Model file for the job. Use its own axes, mm. A direction names the side the tool comes from. Coordinates: 2 decimals unless noted, no trailing zeros. Loops run counter-clockwise (first coordinate to the right, second up) from the corner with the lowest first, then second, coordinate; pieces in that order, holes last. Notation, with made-up numbers: (7, -30) - (33, -30) arc R16 ccw to (33, -22) - close; hole circle Ø5 at (85, 72). An arc over 180 degrees is marked (long way). Write each question's results on one line, items separated by ' | '. Start each with the question number.
```python
from build123d import *

# Parameters (mm, degrees)
F0_W     = 44.45
F0_H     = 228.6
F1_DEPTH = 6.35
F3_DEPTH = 44.45
F5_DEPTH = 12.7
F7_DEPTH = 25.4


with BuildPart() as f1:
    # F0 (on Top) → F1 (new body)
    with BuildSketch(Plane.XY):
        with Locations((0, -114.3)):
            Rectangle(F0_W, F0_H)
    extrude(amount=-F1_DEPTH)

    # F2 (on face) → F3 (join)
    with BuildSketch(Plane.YZ.offset(22.225)):
        with BuildLine():
            ThreePointArc((-21.82495, 0), (-21.592466, -0.561266), (-21.0312, -0.79375))
            Line((-21.0312, -0.79375), (-21.0312, 0))
            Line((-21.0312, 0), (-21.82495, 0))
        make_face()
        with BuildLine():
            Line((-21.0312, 0), (-21.0312, -0.79375))
            ThreePointArc((-21.0312, -0.79375), (-20.469934, -0.561266), (-20.23745, 0))
            Line((-20.23745, 0), (-21.0312, 0))
        make_face()
        with BuildLine():
            ThreePointArc((-41.66235, 0), (-41.429866, -0.561266), (-40.8686, -0.79375))
            Line((-40.8686, -0.79375), (-40.8686, 0))
            Line((-40.8686, 0), (-41.66235, 0))
        make_face()
        with BuildLine():
            Line((-40.8686, 0), (-40.8686, -0.79375))
            ThreePointArc((-40.8686, -0.79375), (-40.307334, -0.561266), (-40.07485, 0))
            Line((-40.07485, 0), (-40.8686, 0))
        make_face()
        with BuildLine():
            ThreePointArc((-60.40755, 0), (-60.175066, -0.561266), (-59.6138, -0.79375))
            Line((-59.6138, -0.79375), (-59.6138, 0))
            Line((-59.6138, 0), (-60.40755, 0))
        make_face()
        with BuildLine():
            Line((-59.6138, 0), (-59.6138, -0.79375))
            ThreePointArc((-59.6138, -0.79375), (-59.052534, -0.561266), (-58.82005, 0))
            Line((-58.82005, 0), (-59.6138, 0))
        make_face()
        with BuildLine():
            ThreePointArc((-78.08595, 0), (-77.853466, -0.561266), (-77.2922, -0.79375))
            Line((-77.2922, -0.79375), (-77.2922, 0))
            Line((-77.2922, 0), (-78.08595, 0))
        make_face()
        with BuildLine():
            Line((-77.2922, 0), (-77.2922, -0.79375))
            ThreePointArc((-77.2922, -0.79375), (-76.730934, -0.561266), (-76.49845, 0))
            Line((-76.49845, 0), (-77.2922, 0))
        make_face()
        with BuildLine():
            ThreePointArc((-94.77375, 0), (-94.541266, -0.561266), (-93.98, -0.79375))
            Line((-93.98, -0.79375), (-93.98, 0))
            Line((-93.98, 0), (-94.77375, 0))
        make_face()
        with BuildLine():
            Line((-93.98, 0), (-93.98, -0.79375))
            ThreePointArc((-93.98, -0.79375), (-93.418734, -0.561266), (-93.18625, 0))
            Line((-93.18625, 0), (-93.98, 0))
        make_face()
        with BuildLine():
            ThreePointArc((-110.52175, 0), (-110.289266, -0.561266), (-109.728, -0.79375))
            Line((-109.728, -0.79375), (-109.728, 0))
            Line((-109.728, 0), (-110.52175, 0))
        make_face()
        with BuildLine():
            Line((-109.728, 0), (-109.728, -0.79375))
            ThreePointArc((-109.728, -0.79375), (-109.166734, -0.561266), (-108.93425, 0))
            Line((-108.93425, 0), (-109.728, 0))
        make_face()
        with BuildLine():
            ThreePointArc((-125.40615, 0), (-125.173666, -0.561266), (-124.6124, -0.79375))
            Line((-124.6124, -0.79375), (-124.6124, 0))
            Line((-124.6124, 0), (-125.40615, 0))
        make_face()
        with BuildLine():
            Line((-124.6124, 0), (-124.6124, -0.79375))
            ThreePointArc((-124.6124, -0.79375), (-124.051134, -0.561266), (-123.81865, 0))
            Line((-123.81865, 0), (-124.6124, 0))
        make_face()
        with BuildLine():
            ThreePointArc((-139.42695, 0), (-139.194466, -0.561266), (-138.6332, -0.79375))
            Line((-138.6332, -0.79375), (-138.6332, 0))
            Line((-138.6332, 0), (-139.42695, 0))
        make_face()
        with BuildLine():
            Line((-138.6332, 0), (-138.6332, -0.79375))
            ThreePointArc((-138.6332, -0.79375), (-138.071934, -0.561266), (-137.83945, 0))
            Line((-137.83945, 0), (-138.6332, 0))
        make_face()
        with BuildLine():
            ThreePointArc((-152.68575, 0), (-152.453266, -0.561266), (-151.892, -0.79375))
            Line((-151.892, -0.79375), (-151.892, 0))
            Line((-151.892, 0), (-152.68575, 0))
        make_face()
        with BuildLine():
            Line((-151.892, 0), (-151.892, -0.79375))
            ThreePointArc((-151.892, -0.79375), (-151.330734, -0.561266), (-151.09825, 0))
            Line((-151.09825, 0), (-151.892, 0))
        make_face()
        with BuildLine():
            ThreePointArc((-165.18255, 0), (-164.950066, -0.561266), (-164.3888, -0.79375))
            Line((-164.3888, -0.79375), (-164.3888, 0))
            Line((-164.3888, 0), (-165.18255, 0))
        make_face()
        with BuildLine():
            Line((-164.3888, 0), (-164.3888, -0.79375))
            ThreePointArc((-164.3888, -0.79375), (-163.827534, -0.561266), (-163.59505, 0))
            Line((-163.59505, 0), (-164.3888, 0))
        make_face()
        with BuildLine():
            ThreePointArc((-176.96815, 0), (-176.735666, -0.561266), (-176.1744, -0.79375))
            Line((-176.1744, -0.79375), (-176.1744, 0))
            Line((-176.1744, 0), (-176.96815, 0))
        make_face()
        with BuildLine():
            Line((-176.1744, 0), (-176.1744, -0.79375))
            ThreePointArc((-176.1744, -0.79375), (-175.613134, -0.561266), (-175.38065, 0))
            Line((-175.38065, 0), (-176.1744, 0))
        make_face()
        with BuildLine():
            ThreePointArc((-188.11875, 0), (-187.886266, -0.561266), (-187.325, -0.79375))
            Line((-187.325, -0.79375), (-187.325, 0))
            Line((-187.325, 0), (-188.11875, 0))
        make_face()
        with BuildLine():
            Line((-187.325, 0), (-187.325, -0.79375))
            ThreePointArc((-187.325, -0.79375), (-186.763734, -0.561266), (-186.53125, 0))
            Line((-186.53125, 0), (-187.325, 0))
        make_face()
        with BuildLine():
            Line((-40.8686, 0), (-40.07485, 0))
            ThreePointArc((-40.07485, 0), (-40.8686, 0.79375), (-41.66235, 0))
            Line((-41.66235, 0), (-40.8686, 0))
        make_face()
        with BuildLine():
            Line((-59.6138, 0), (-58.82005, 0))
            ThreePointArc((-58.82005, 0), (-59.6138, 0.79375), (-60.40755, 0))
            Line((-60.40755, 0), (-59.6138, 0))
        make_face()
        with BuildLine():
            Line((-77.2922, 0), (-76.49845, 0))
            ThreePointArc((-76.49845, 0), (-77.2922, 0.79375), (-78.08595, 0))
            Line((-78.08595, 0), (-77.2922, 0))
        make_face()
        with BuildLine():
            Line((-93.98, 0), (-93.18625, 0))
            ThreePointArc((-93.18625, 0), (-93.98, 0.79375), (-94.77375, 0))
            Line((-94.77375, 0), (-93.98, 0))
        make_face()
        with BuildLine():
            Line((-109.728, 0), (-108.93425, 0))
            ThreePointArc((-108.93425, 0), (-109.728, 0.79375), (-110.52175, 0))
            Line((-110.52175, 0), (-109.728, 0))
        make_face()
        with BuildLine():
            Line((-124.6124, 0), (-123.81865, 0))
            ThreePointArc((-123.81865, 0), (-124.6124, 0.79375), (-125.40615, 0))
            Line((-125.40615, 0), (-124.6124, 0))
        make_face()
        with BuildLine():
            Line((-138.6332, 0), (-137.83945, 0))
            ThreePointArc((-137.83945, 0), (-138.6332, 0.79375), (-139.42695, 0))
            Line((-139.42695, 0), (-138.6332, 0))
        make_face()
        with BuildLine():
            Line((-151.892, 0), (-151.09825, 0))
            ThreePointArc((-151.09825, 0), (-151.892, 0.79375), (-152.68575, 0))
            Line((-152.68575, 0), (-151.892, 0))
        make_face()
        with BuildLine():
            Line((-164.3888, 0), (-163.59505, 0))
            ThreePointArc((-163.59505, 0), (-164.3888, 0.79375), (-165.18255, 0))
            Line((-165.18255, 0), (-164.3888, 0))
        make_face()
        with BuildLine():
            Line((-176.1744, 0), (-175.38065, 0))
            ThreePointArc((-175.38065, 0), (-176.1744, 0.79375), (-176.96815, 0))
            Line((-176.96815, 0), (-176.1744, 0))
        make_face()
        with BuildLine():
            Line((-187.325, 0), (-186.53125, 0))
            ThreePointArc((-186.53125, 0), (-187.325, 0.79375), (-188.11875, 0))
            Line((-188.11875, 0), (-187.325, 0))
        make_face()
        with BuildLine():
            Line((-21.82495, 0), (-21.0312, 0))
            Line((-21.0312, 0), (-20.23745, 0))
            ThreePointArc((-20.23745, 0), (-21.0312, 0.79375), (-21.82495, 0))
        make_face()
    extrude(amount=-F3_DEPTH)

    # F4 (on Top) → F5 (cut, symmetric)
    with BuildSketch(Plane.XY):
        Polygon((22.286486, 0), (14.2875, 0), (22.286486, -228.6), align=None)
        Polygon((-14.2875, 0), (-22.363186, 0), (-22.363186, -228.6), align=None)
    extrude(amount=F5_DEPTH, both=True, mode=Mode.SUBTRACT)

    # F6 (on face) → F7 (cut)
    with BuildSketch(Plane.XY):
        with BuildLine():
            Line((-22.225, -228.6), (22.225, -228.6))
            ThreePointArc((22.225, -228.6), (0, -222.991998), (-22.225, -228.6))
        make_face()
    extrude(amount=-F7_DEPTH, mode=Mode.SUBTRACT)


solid = f1.part
```
Q1. Mould opens along Y. For faces 1 (the flat face through (0, -113, -6.35)), 2 (the flat face through (0, 0, -3)), 3 (the flat face through (0, -158, 0)), 4 (the cylindrical face through (0.324, -222.993, -3.131)) say: +Y half, -Y half, draft (parallel to the pull), parting line (faces both ways), or undercut.
Q2. Cut at A-A (z = -3). List the corners of the cut face in (x, y) (1 decimal), and give its area (3 significant figures).
Q3. Pin check, flat tip, straight feed: pin 1 (12 mm diameter, centred on x = -6.5, y = -206, fed in from +Z). Stop position of the tip, or through.
Q4. Cut at C-C (y = -204). List the corners of the cut face in (x, z), and give its area (3 significant figures).
Q5. Which spindle directions (+Z, -Z, +X, -X, +Y, -Y) get a long thin tool onto all of the face, cutting with end or side? Do faces 5 (the flat face through (0, -10, 0)), 6 (the flat face through (0, -208, 0)), 7 (the flat face through (0, -86, 0)). Say none if no direction does.
Q6. Drill centre lines: L1, parallel to Z at x = 15, y = -118; L2, parallel to Z at x = -11, y = -41; L3, parallel to X at y = -77, z = -2.5. Where is each one in solid material? Low to high. Write a range as from..to.
Check result:
1) face 1: draft | face 2: +Y half | face 3: undercut | face 4: -Y half
2) outline: (-22.2, -228.6) arc R46.8 cw to (22.2, -228.6) - (22.2, -226.8) - (14.3, 0) - (-14.3, 0) - (-22.2, -224.7) - close | area: 8,200 mm²
3) pin 1: z = 0
4) outline: (-21.49, -6.35) - (21.43, -6.35) - (21.43, 0) - (-21.49, 0) - close | area: 273 mm²
5) face 5: +Z, +X, -X, +Y | face 6: +Z, +X, -X, -Y | face 7: +Z, +X, -X
6) L1: -6.35..0 | L2: -6.35..0.78 | L3: -17.01..16.98
